```python
from build123d import *

# Parameters (mm, degrees)
F0_W     = 82.55
F0_H     = 88.9
F1_DEPTH = 12.7
F3_D     = 38.1
F4_W     = 5.5692129374
F4_H     = 88.9
F5_DEPTH = 38.1
F6_W     = 88.9
F6_H     = 38.1
F7_DEPTH = 23.6223284155


with BuildPart() as f1:
    # F0 (on Top) → F1 (new body)
    with BuildSketch(Plane.XY):
        with Locations((41.275, -44.45)):
            Rectangle(F0_W, F0_H)
        with Locations((123.825, -44.45)):
            Rectangle(F0_W, F0_H)
    extrude(amount=F1_DEPTH)

    # F3 (through all)
    with Locations(Plane(origin=(0, 0, 0), x_dir=(1, 0, 0), z_dir=(0, 0, -1))):
        with Locations((123.825, 44.45), (41.275, 44.45)):
            Hole(F3_D / 2)

    # F4 (on face) → F5 (join)
    with BuildSketch(Plane(origin=(0, 0, 0), x_dir=(1, 0, 0), z_dir=(0, 0, -1))):
        with Locations((167.8846064687, 44.45)):
            Rectangle(F4_W, F4_H)
    extrude(amount=-F5_DEPTH)

    # F6 (on face) → F7 (join)
    with BuildSketch(Plane.YZ.offset(170.6692129374)):
        with Locations((-44.45, 19.05)):
            Rectangle(F6_W, F6_H)
    extrude(amount=F7_DEPTH)


solid = f1.part
```
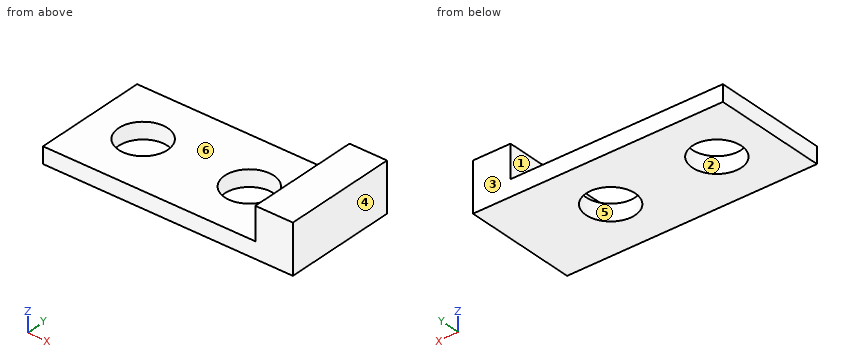
Check sheet for the modelled part. Datum: model origin and axes. Units: mm. Face numbers are marked on the shaded views. A direction names the side the tool comes from. Give positions to 0.01 mm unless a question says otherwise; leave off trailing zeros. Loops run counter-clockwise (first coordinate to the right, second up) from the corner with the lowest first, then second, coordinate; pieces in that order, holes last. Notation, with made-up numbers: M 72.5,2 L 108.5,2 A29 ccw 108.5,30 Z; hole C 5,60 d7. An arc over 180 degrees is marked long. Answer as CSV lines item,"result".
Item 1: Depth check by flat-ended pin: pin 1 Ø10 at (y, z) = (-40.5, 24.5) entering from -X; pin 2 Ø10 at (x, y) = (83, -73.5) entering from +Z. Enter the tip coordinate at first touch or a pass-through.
Reply:
pin 1,"x = 165.1"
pin 2,"z = 12.7"
Item 2: Sectioned sample at C-C, the plane x = 28.5. Enter the section's corners in (y, z), then the cut area to 3 significant figures.
Reply:
outline,"M -88.9,0 L -58.58,0 L -58.58,12.7 L -88.9,12.7 Z; M -30.32,0 L 0,0 L 0,12.7 L -30.32,12.7 Z"
area,"770 mm^2"
Item 3: Set-up check for the marked faces 5 and 6: record each of +Z, -Z, +X, -X, +Y, -Y from which the full face is reachable in a straight line by a thin tool's end or side.
Reply:
face 5,"+Z, -Z"
face 6,"+Z, -X, +Y, -Y"
Item 4: Sectioned sample at A-A, the plane y = -44.45. Enter the section's corners in (x, z) (3 decimals).
Reply:
outline,"M 0,0 L 22.225,0 L 22.225,12.7 L 0,12.7 Z; M 60.325,0 L 104.775,0 L 104.775,12.7 L 60.325,12.7 Z; M 142.875,0 L 194.292,0 L 194.292,38.1 L 165.1,38.1 L 165.1,12.7 L 142.875,12.7 Z"
Item 5: Sectioned sample at D-D, the plane y = -21.5. Enter the section's corners in (x, z).
Reply:
outline,"M 0,0 L 194.29,0 L 194.29,38.1 L 165.1,38.1 L 165.1,12.7 L 0,12.7 Z"
Item 6: Sectioned sample at B-B, the plane z = 5. Enter the section's corners in (x, y) (3 decimals), then the cut area to 3 significant figures.
Reply:
outline,"M 0,-88.9 L 194.292,-88.9 L 194.292,0 L 0,0 Z; hole C 41.275,-44.45 d38.1; hole C 123.825,-44.45 d38.1"
area,"15,000 mm^2"
Item 7: Scan lines: L1, parallel to Z at x = 71.5, y = -11; L2, parallel to Y at x = 133.5, z = 3.5; L3, parallel to Y at x = 25.5, z = 2. Record each from-to range of solid material in increasing order.
Reply:
L1,"0 to 12.7"
L2,"-88.9 to -60.86, -28.04 to 0"
L3,"-88.9 to -55.13, -33.77 to 0"
Item 8: Draft check along X on the marked faces 1, 2, 3 and 4. Enter one of: pulls with the +X half, pulls with the -X half, needs draft (parallel to the pull), parting line crosses it, or undercut.
Reply:
face 1,"pulls with the -X half"
face 2,"undercut"
face 3,"needs draft"
face 4,"pulls with the +X half"
